Model file for the job. Use its own axes, mm. Coordinates: 2 decimals unless noted, no trailing zeros. Order: outer loops, then holes, each group sorted by start corner. A loop starts at its lowest first (then second) coordinate and runs counter-clockwise, first axis right, second up. Notation, with made-up numbers: M -40,-19 L 18,-19 A29 cw 18,15 Z; hole C 84.25,72 d8. An arc over 180 degrees is marked long. Return JSON: item names as keys, results as strings.
```python
from build123d import *

# Parameters (mm, degrees)
F0_W     = 44.45
F0_H     = 50.8
F1_DEPTH = 12.7
F2_SIZE  = 5.08
F4_D     = 1.27


with BuildPart() as f1:
    # F0 (on Top) → F1 (new body)
    with BuildSketch(Plane.XY):
        with Locations((-22.886127, -14.839125)):
            Rectangle(F0_W, F0_H)
    extrude(amount=F1_DEPTH)

    # F2
    f2_edges = [f1.edges().sort_by_distance(p)[0] for p in [
        (-45.111127, -14.839125, 12.7),
        (-22.886127, -40.239125, 12.7),
        (-0.661127, -14.839125, 12.7),
        (-22.886127, 10.560875, 12.7),
        (-45.111127, -14.839125, 0),
        (-22.886127, -40.239125, 0),
        (-0.661127, -14.839125, 0),
        (-0.661127, 10.560875, 6.35),
        (-45.111127, 10.560875, 6.35),
        (-22.886127, 10.560875, 0),
        (-0.661127, -40.239125, 6.35),
        (-45.111127, -40.239125, 6.35),
    ]]
    chamfer(f2_edges, length=F2_SIZE)

    # F4 (through all)
    with Locations(Plane.XZ.offset(40.239125)):
        with Locations((-38.692214, 6.35)):
            Hole(F4_D / 2)


solid = f1.part
```
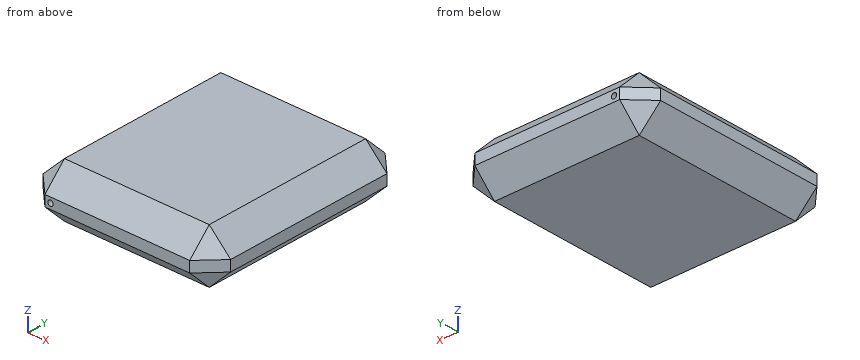
Item 1: Drop flat-ended pins along their axis: pin 1 Ø2 at (y, z) = (-4, 1.5) entering from -X; pin 2 Ø3 at (y, z) = (4, 8) entering from -X; pin 3 Ø1 at (y, z) = (-5.5, 11) entering from +X; pin 4 Ø5 at (x, z) = (-31.5, 2.5) entering from +Y. Give the stop position or say it passes through.
Check result:
{"pin 1": "stops at x = -42.53", "pin 2": "stops at x = -45.11", "pin 3": "stops at x = -3.54", "pin 4": "stops at y = 10.48"}
Item 2: Saw through at C-C (x = -20.5). Write the cut outline in (y, z).
Check result:
{"outline": "M -40.24,5.08 L -35.16,0 L 5.48,0 L 10.56,5.08 L 10.56,7.62 L 5.48,12.7 L -35.16,12.7 L -40.24,7.62 Z"}
Item 3: Saw through at B-B (z = 6.35). Write the cut outline in (x, y).
Check result:
{"outline": "M -45.11,-35.16 L -40.03,-40.24 L -39.33,-40.24 L -39.33,10.56 L -40.03,10.56 L -45.11,5.48 Z; M -38.06,-40.24 L -5.74,-40.24 L -0.66,-35.16 L -0.66,5.48 L -5.74,10.56 L -38.06,10.56 Z"}
Item 4: Saw through at A-A (y = 4). Write the cut outline in (x, z) (3 decimals), and give its area (3 significant figures).
Check result:
{"outline": "M -45.111,5.08 L -40.031,0 L -5.741,0 L -0.661,5.08 L -0.661,7.62 L -5.741,12.7 L -40.031,12.7 L -45.111,7.62 Z; hole C -38.692,6.35 d1.27", "area": "512 mm2"}
Item 5: Saw through at D-D (x = -3.5). Write the cut outline in (y, z), and give its area (3 significant figures).
Check result:
{"outline": "M -38,5.08 L -35.16,2.24 L 5.48,2.24 L 8.32,5.08 L 8.32,7.62 L 5.48,10.46 L -35.16,10.46 L -38,7.62 Z", "area": "365 mm2"}
Item 6: Wall check: line 1 (X direction, y = 3.5, z = 6.5); line 2 (Z direction, x = -14.5, y = 6.5); line 3 (X direction, y = 0, z = 0.75). Give the ranges that are in metal, low to high.
Check result:
{"line 1": "x = -45.11 to -39.31, -38.08 to -0.66", "line 2": "z = 1.02 to 11.68", "line 3": "x = -40.78 to -4.99"}
